```python
from build123d import *

# Parameters (mm, degrees)
EXTRUDE_1_DEPTH          = 95
SKETCH_2_R               = 1.5
CUT_EXTRUDE_1_DEPTH      = 12.002837415
CUT_EXTRUDE_1_DEPTH_BACK = 3.00301723
CUT_EXTRUDE_2_DEPTH      = 14.002837554


with BuildPart() as part:
    # Эскиз1 → Бобышка-Вытянуть1 (new body)
    with BuildSketch(Plane(origin=(0, 0, 0), x_dir=(0, 0, -1), z_dir=(1, 0, 0))):
        with BuildLine():
            Line((11, 0), (18.079487192, 0))
            Line((18.079487192, 0), (18.079487192, 2))
            Line((18.079487192, 2), (12.848104212, 2))
            ThreePointArc((12.848104212, 2), (0.000220895, 13.002837452), (-12.848036252, 2.000436531))
            Line((-12.848036252, 2.000436531), (-18.079487192, 2))
            Line((-18.079487192, 2), (-18.079487192, 0))
            Line((-18.079487192, 0), (-11, 0))
            ThreePointArc((-11, 0), (0, 11), (11, 0))
        make_face()
    extrude(amount=EXTRUDE_1_DEPTH)

    # Эскиз2 → Вырез-Вытянуть1 (cut, two sides)
    with BuildSketch(Plane(origin=(0, 2.001508604, 0.000167013), x_dir=(1, 0, 0), z_dir=(0, 0.999999997, 8.3444e-05))) as cut_extrude_1_sk:
        with Locations((27.5, -16)):
            Circle(SKETCH_2_R)
        with Locations((67.5, -16)):
            Circle(SKETCH_2_R)
        with Locations((67.5, 16)):
            Circle(SKETCH_2_R)
        with Locations((27.5, 16)):
            Circle(SKETCH_2_R)
        with BuildLine():
            Line((4.5, -14.579320241), (4.5, -18.29882224))
            Line((4.5, -18.29882224), (10.5, -18.29882224))
            Line((10.5, -18.29882224), (10.5, -14.579320241))
            ThreePointArc((10.5, -14.579320241), (7.5, -11.579320241), (4.5, -14.579320241))
        make_face()
        with BuildLine():
            Line((50.5, -18.29882224), (50.5, -14.579320241))
            ThreePointArc((50.5, -14.579320241), (47.5, -11.579320241), (44.5, -14.579320241))
            Line((44.5, -14.579320241), (44.5, -18.29882224))
            Line((44.5, -18.29882224), (50.5, -18.29882224))
        make_face()
        with BuildLine():
            Line((90.5, -18.29882224), (90.5, -14.579320241))
            ThreePointArc((90.5, -14.579320241), (87.5, -11.579320241), (84.5, -14.579320241))
            Line((84.5, -14.579320241), (84.5, -18.29882224))
            Line((84.5, -18.29882224), (90.5, -18.29882224))
        make_face()
        with BuildLine():
            Line((84.5, 18.29882224), (90.5, 18.29882224))
            Line((90.5, 18.29882224), (90.5, 14.579320241))
            ThreePointArc((90.5, 14.579320241), (87.5, 11.579320241), (84.5, 14.579320241))
            Line((84.5, 14.579320241), (84.5, 18.29882224))
        make_face()
        with BuildLine():
            Line((44.5, 18.29882224), (50.5, 18.29882224))
            Line((50.5, 18.29882224), (50.5, 14.579320241))
            ThreePointArc((50.5, 14.579320241), (47.5, 11.579320241), (44.5, 14.579320241))
            Line((44.5, 14.579320241), (44.5, 18.29882224))
        make_face()
        with BuildLine():
            Line((4.5, 18.29882224), (10.5, 18.29882224))
            Line((10.5, 18.29882224), (10.5, 14.579320241))
            ThreePointArc((10.5, 14.579320241), (7.5, 11.579320241), (4.5, 14.579320241))
            Line((4.5, 14.579320241), (4.5, 18.29882224))
        make_face()
    extrude(amount=CUT_EXTRUDE_1_DEPTH, mode=Mode.SUBTRACT)
    extrude(cut_extrude_1_sk.sketch, amount=-CUT_EXTRUDE_1_DEPTH_BACK, mode=Mode.SUBTRACT)

    # Эскиз3 → Вырез-Вытянуть2 (cut, through all)
    with BuildSketch(Plane.XZ):
        with BuildLine():
            Line((85.409616901, 5), (95, 5))
            Line((95, 5), (95, -5))
            Line((95, -5), (85.409616901, -5))
            ThreePointArc((85.409616901, -5), (82.227636386, -3.681980515), (80.909616901, -0.5))
            Line((80.909616901, -0.5), (80.909616901, 0.5))
            ThreePointArc((80.909616901, 0.5), (82.227636386, 3.681980515), (85.409616901, 5))
        make_face()
    extrude(amount=-CUT_EXTRUDE_2_DEPTH, mode=Mode.SUBTRACT)


solid = part.part
```
Can you work these out from the model? Positions are in its coordinate system, mm. A direction names the side the tool comes from. Coordinates: 2 decimals unless noted, no trailing zeros. Write each loop counter-clockwise with the first axis right and the second up, starting at its lowest first coordinate (ties: lowest second). Pieces come first, ordered by that corner, then holes. Notation, with made-up numbers: M 56,35 L 67,35 A7 ccw 67,42 Z; hole C 14,2 d2. An arc over 180 degrees is marked long. Write item = value, one per line. Start each with the question number.
Q1. On a 3-axis mill with a long thin cutter (end or side, diameter ignored), from which of +Z, -Z, +X, -X, +Y, -Y can I reach the whole of each face in a straight line? I mean faces 5 (the face through (92, 2, -16)), 6 (the face through (93, 1, -18.079)), 7 (the face through (67, 1, 18.079)), 8 (the face through (50.5, 1, -16)), 9 (the face through (4.5, 1, 16)). Say none if no direction works.
Q2. If I drill on L1, parallel to Z at x = 27.5, y = 0.55; L2, parallel to Z at x = 28, y = 1.75; L3, parallel to Y at x = 81, z = 16.5, over which ranges is the centre line in solid material (lowest first)? Write a range as [from, to].
Q3. If we section it at A-A, the plane x = 27.5: Write out the boundary of the cut face in (y, z).
Q4. I'm going to push flat-ended pins straight in: pin 1 (5 mm diameter, centred on y = 9, z = 1.5, fed in from +X); pin 2 (10 mm diameter, centred on x = 80.5, z = 5.5, fed in from +Y); pin 3 (2.5 mm diameter, centred on x = 67.5, z = 16, fed in from +Y); pin 4 (1.8 mm diameter, centred on x = 91, y = 11, fed in from +Z). Where does each tip first touch, or does it pass through?
Q5. If we section it at B-B, the plane x = 87.5: Write out the boundary of the cut face in (y, z), then the cut area to 3 significant figures.
Q6. If we section it at C-C, the plane x = 7.5: Write out the boundary of the cut face in (y, z), then the cut area to 3 significant figures.
Q7. Thinking about a two-plate mould opening in Z: for faces 1 (the face through (26, 1, 16)), 2 (the face through (47, 11, 0)), 3 (the face through (90.5, 1, -16)), 4 (the face through (93, 1, 18.079)), which applies, released by +Z, released by -Z, zero draft, split by the parting line, or undercut?
Check sheet entries:
q1.face_5 = -Z, +X, -X, +Y
q1.face_6 = -Z, +X, -X, +Y, -Y
q1.face_7 = +Z, +X, -X, +Y, -Y
q1.face_8 = -Z, +Y, -Y
q1.face_9 = +Z, +Y, -Y
q2.L1 = [-18.08, -17.5], [-14.5, -10.99], [10.99, 14.5], [17.5, 18.08]
q2.L2 = [-18.08, -17.41], [-14.59, -10.86], [10.86, 14.59], [17.41, 18.08]
q2.L3 = [0, 2]
q3.outline = M 0,-18.08 L 2,-18.08 L 2,-17.5 L 0,-17.5 Z; M 0,-14.5 L 2,-14.5 L 2,-12.85 A13 ccw 2,12.85 L 2,14.5 L 0,14.5 L 0,11 A11 cw 0,-11 Z; M 0,17.5 L 2,17.5 L 2,18.08 L 0,18.08 Z
q4.pin_1 = 82.12
q4.pin_2 = 12.99
q4.pin_3 = through
q4.pin_4 = 8.19
q5.outline = M 0,-11.58 L 5.92,-11.58 A13 ccw 12,-5 L 9.8,-5 A11 cw 0,-11 Z; M 0,11 A11 cw 9.8,5 L 12,5 A13 ccw 5.91,11.58 L 0,11.58 Z
q5.area = 43.5 mm²
q6.outline = M 0,-11.58 L 5.92,-11.58 A13 ccw 5.91,11.58 L 0,11.58 L 0,11 A11 cw 0,-11 Z
q6.area = 64.2 mm²
q7.face_1 = undercut
q7.face_2 = undercut
q7.face_3 = zero draft
q7.face_4 = released by +Z
